For this review, take the finished solid that the model builds, in its own axes (mm). Give positions to 0.01 mm unless a question says otherwise; leave off trailing zeros. Order: outer loops, then holes, each group sorted by start corner. A loop starts at its lowest first (then second) coordinate and runs counter-clockwise, first axis right, second up. Notation, with made-up numbers: M 6,19.25 L 44,19.25 A19 ccw 44,26.25 Z; hole C -4,84 d3. An arc over 180 degrees is marked long. Answer as CSV lines item,"result". Start each with the question number.
1. We need section B-B, the plane y = -6. Give the boundary of the cut face in (x, z), and give its area (3 significant figures).
2. For line 1 along X through (y, z) = (6.75, 6.25); line 2 along X through (y, z) = (4.25, 6.25); line 3 along Y through (x, z) = (-27, 1.5), list the stretches that pass through material, from the lowest coordinate up.
3. We need section C-C, the plane x = -21.5. Give the boundary of the cut face in (y, z), and give its area (3 significant figures).
4. We need section A-A, the plane z = 5.5. Give the boundary of the cut face in (x, y).
from build123d import *

# Parameters (mm, degrees)
F0_W     = 10
F0_H     = 5
F1_DEPTH = 7


with BuildPart() as f1:
    # F0 (on Top) → F1 (new body)
    with BuildSketch(Plane.XY):
        Polygon((-20, -7.5), (20, -7.5), (20, 7.5), (-20, 7.5), (-20, 2.5), (-20, -2.5), align=None)
        Polygon((-30, -2.5), (-20, -7.5), (-20, -2.5), align=None)
        with Locations((-25, 0)):
            Rectangle(F0_W, F0_H)
        Polygon((-20, 2.5), (-20, 7.5), (-30, 2.5), align=None)
    extrude(amount=F1_DEPTH)


solid = f1.part
Result set:
1,outline,"M -23,0 L 20,0 L 20,7 L -23,7 Z"
1,area,"301 mm2"
2,line 1,"-21.5 to 20"
2,line 2,"-26.5 to 20"
2,line 3,"-4 to 4"
3,outline,"M -6.75,0 L 6.75,0 L 6.75,7 L -6.75,7 Z"
3,area,"94.5 mm2"
4,outline,"M -30,-2.5 L -20,-7.5 L 20,-7.5 L 20,7.5 L -20,7.5 L -30,2.5 Z"
